Autodesk Inventor part; units mm, degrees
ref_plane "YZ Plane" through (0, 0, 0) normal (1, 0, 0) x (0, 1, 0)
ref_plane "XZ Plane" through (0, 0, 0) normal (0, 1, 0) x (-1, 0, 0)
ref_plane "XY Plane" through (0, 0, 0) normal (0, 0, 1) x (1, 0, 0)
sketch "スケッチ1" plane through (0, 0, 0) normal (0, 0, 1) x (1, 0, 0)
  line L0 (30, 0) -> (30, 350)
  line L1 (0, 350) -> (0, 0)
  arc A0 (30, 350) -> (0, 350) centre (15, 350) ccw
  arc A1 (0, 0) -> (30, 0) centre (15, 0) ccw
  dimension "d35" = 30
  dimension "d36" = 350
extrude "押し出し1" add sketch "スケッチ1" along normal blind 2
sketch "スケッチ3" plane through (0, 0, 2) normal (0, 0, 1) x (1, 0, 0)
  line L0 (0, 350) -> (0, 0)
  arc A0 (0, 0) -> (30, 0) centre (15, 0) ccw
  line L1 (0, 0) -> (30, 0) construction
  point P0 (7.5, 0)
  point P1 (15, -7.5)
  point P2 (22.5, 0)
  point P3 (15, 7.5)
  dimension "d41" = 7.5
  dimension "d44" = 360
hole "穴1" at (7.5, 0, 2) at (15, -7.5, 2) at (22.5, 0, 2) at (15, 7.5, 2) direction (0, 0, -1) diameter 2.8 end through all
properties part number "arm_link" material "GFRP"
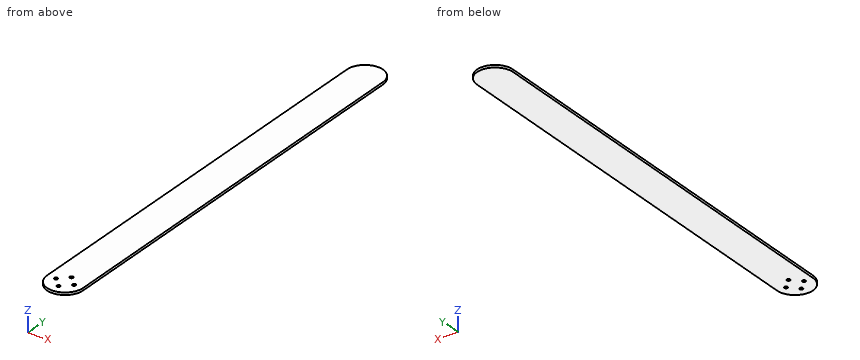
Geometry: final body of the model. Coordinates: model frame, mm. Coordinates: 2 decimals unless noted, no trailing zeros. Order: outer loops, then holes, each group sorted by start corner. A loop starts at its lowest first (then second) coordinate and runs counter-clockwise, first axis right, second up. Notation, with made-up numbers: (-38.5, 47) - (-33.5, 47) arc R8 ccw to (-33.5, 51) - close; hole circle Ø3 at (47, 1.5). An arc over 180 degrees is marked (long way). Return JSON: item names as keys, results as strings. Group by question number.
1. Material intervals for line 1 along X through (y, z) = (0, 1.55); line 2 along Y through (x, z) = (15, 0.8); line 3 along X through (y, z) = (7.5, 0.6), sorted ascending. Write a range as [from, to].
2. Cut plane A-A (z = 1). Output: boundary loops of the cut face in (x, y).
3. Pin query (flat end, axial travel): pin 1 (8 mm diameter, centred on x = 6, y = 41.5, fed in from -Z); pin 2 (2.5 mm diameter, centred on x = 15, y = 7.5, fed in from -Z). Return the tip coordinate at first contact, or that it passes through.
Resolved:
{
 "1": {"line 1": "x = [0, 6.1], [8.9, 21.1], [23.9, 30]", "line 2": "y = [-15, -8.9], [-6.1, 6.1], [8.9, 365]", "line 3": "x = [0, 13.6], [16.4, 30]"},
 "2": {"outline": "(0, 0) arc R15 ccw to (30, 0) - (30, 350) arc R15 ccw to (0, 350) - close; hole circle Ø2.8 at (7.5, 0); hole circle Ø2.8 at (15, -7.5); hole circle Ø2.8 at (15, 7.5); hole circle Ø2.8 at (22.5, 0)"},
 "3": {"pin 1": "stops at z = 0", "pin 2": "passes through"}
}
